Autodesk Fusion 360 part; units mm, degrees
sketch "Sketch1" plane through (0, 0, 0) normal (0, 0, 1) x (1, 0, 0)
  line L0 (0, 25) -> (64, 25)
  line L1 (64, 25) -> (64, -13)
  line L2 (64, -13) -> (0, -13)
  line L3 (0, -13) -> (0, 25)
  dimension "d1" = 64
  dimension "d2" = 38
extrude "Extrude1" add sketch "Sketch1" along normal blind 38
sketch "Sketch2" plane through (0, 0, 38) normal (0, 0, 1) x (1, 0, 0)
  line L0 (0, -13) -> (64, -13)
  line L1 (64, -13) -> (64, 25)
  line L2 (64, 25) -> (0, 25)
  line L3 (0, 25) -> (0, -13)
  line L4 (0, 25) -> (64, -13) construction
  line L5 (40.5159, 20.75) -> (23.4841, 20.75)
  line L6 (23.4841, 20.75) -> (14.9682, 6)
  line L7 (14.9682, 6) -> (23.4841, -8.75)
  line L8 (23.4841, -8.75) -> (40.5159, -8.75)
  line L9 (40.5159, -8.75) -> (49.0318, 6)
  line L10 (49.0318, 6) -> (40.5159, 20.75)
  circle A0 centre (32, 6) radius 11.75
  point P0 (32, 6)
  point P1 (32, 6)
  dimension "d5" = 14.75
  dimension "d8" = 23.5
extrude "Extrude2" cut sketch "Sketch2" against normal blind 8 contours L5 L6 L7 L8 L9 L10 | A0
extrude "Extrude3" cut sketch "Sketch2" against normal blind 52 contours A0
sketch "Sketch4" plane through (0, 0, 0) normal (-1, 0, 0) x (0, 0, 1)
  line L0 (0, 25) -> (0, -13)
  line L1 (0, -13) -> (38, -13)
  line L2 (38, -13) -> (38, 25)
  line L3 (38, 25) -> (0, 25)
  circle A0 centre (19, 6) radius 6.75 construction
  line L4 (2.0294, 22.9706) -> (35.9706, -10.9706) construction
  line L5 (19, 25) -> (19, -13) construction
  line L6 (2.0294, -10.9706) -> (35.9706, 22.9706) construction
  line L7 (2.0294, 22.9706) -> (11.3071, 6)
  line L8 (2.0294, 22.9706) -> (19, 13.6929)
  line L9 (35.9706, 22.9706) -> (19, 13.6929)
  line L10 (35.9706, 22.9706) -> (26.6929, 6)
  line L11 (35.9706, -10.9706) -> (26.6929, 6)
  line L12 (35.9706, -10.9706) -> (19, -1.6929)
  line L13 (2.0294, -10.9706) -> (19, -1.6929)
  line L14 (2.0294, -10.9706) -> (11.3071, 6)
  line L15 (19, 6) -> (2.0294, 22.9706) construction
  line L16 (8.5702, 16.4298) -> (10.5147, 18.3317) construction
  line L17 (9.5, 15.5) -> (11.6895, 17.6895) construction
  line L18 (11.3986, 13.6014) -> (14.1445, 16.3473) construction
  line L19 (12.8128, 12.1872) -> (15.9732, 15.3476) construction
  line L20 (9.5, 15.5) -> (28.5, 15.5) construction
  line L21 (28.5, 15.5) -> (28.5, -3.5) construction
  line L22 (28.5, -3.5) -> (9.5, -3.5) construction
  line L23 (9.5, -3.5) -> (9.5, 15.5) construction
  line L24 (28.5, 15.5) -> (9.5, -3.5) construction
  circle A1 centre (9.5, 15.5) radius 1
  circle A2 centre (28.5, 15.5) radius 1
  circle A3 centre (28.5, -3.5) radius 1
  circle A4 centre (9.5, -3.5) radius 1
  point P0 (19, 6)
  point P1 (12.8128, 12.1872)
  point P2 (11.3986, 13.6014)
  point P3 (9.5, 15.5)
  point P4 (8.5702, 16.4298)
  point P5 (14.227, 10.773)
  point P6 (28.5, 15.5)
  point P7 (9.5, -3.5)
  point P8 (28.5, -3.5)
  dimension "d11" = 13.5
  dimension "d12" = 48
  dimension "d13" = 48
  dimension "d33" = 19
  dimension "d34" = -19
  dimension "d35" = 2
  dimension "d36" = 2
  dimension "d37" = 2
  dimension "d38" = 2
extrude "Extrude4" cut sketch "Sketch4" against normal blind 3 contours L7 L8 L9 L10 L11 L12 L13 L14 | A1 | A2 | A3 | A4
fillet "Fillet1" radius 3 2 edges at (32, 25, 0) (32, -13, 0)
fillet "Fillet2" radius 3 2 edges at (32, 25, 38) (32, -13, 38)
sketch "Sketch5" plane through (64, 0, 0) normal (1, 0, 0) x (0, 0, -1)
  arc A0 (-38, -10) -> (-35, -13) centre (-35, -10) ccw
  line L0 (-35, -13) -> (-3, -13)
  arc A1 (-3, -13) -> (0, -10) centre (-3, -10) ccw
  line L1 (0, -10) -> (0, 22)
  arc A2 (0, 22) -> (-3, 25) centre (-3, 22) ccw
  line L2 (-3, 25) -> (-35, 25)
  arc A3 (-35, 25) -> (-38, 22) centre (-35, 22) ccw
  line L3 (-38, 22) -> (-38, -10)
  circle A4 centre (-19, 6) radius 11.25
  circle A5 centre (-19, 6) radius 4.5
  point P0 (-19, 25)
  point P1 (-19, -13)
  point P2 (-38, 6)
  point P3 (0, 6)
  point P4 (-19, 6)
  dimension "d20" = 22.5
  dimension "d21" = 9
extrude "Extrude5" cut sketch "Sketch5" against normal blind 18 contours A5
extrude "Extrude6" cut sketch "Sketch5" against normal blind 7 contours A4
extrude "Extrude7" cut sketch "Sketch4" against normal blind 4 contours L7 L8 L9 L10 L11 L12 L13 L14 | A1 | A2 | A3 | A4
extrude "Extrude8" cut sketch "Sketch4" against normal blind 7 contours A1 | A2 | A3 | A4
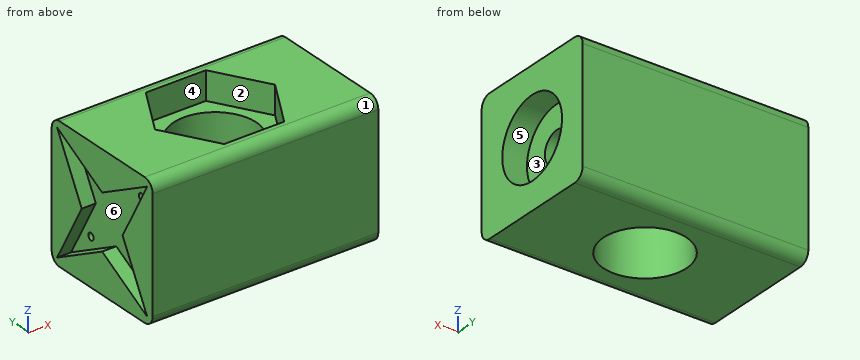
Geometry: final body of the model. Coordinates: model frame, mm. Face numbers are marked on the shaded views. A direction names the side the tool comes from. Coordinates: 2 decimals unless noted, no trailing zeros. Order: outer loops, then holes, each group sorted by start corner. A loop starts at its lowest first (then second) coordinate and runs counter-clockwise, first axis right, second up. Notation, with made-up numbers: M -23.75,51 L -12.75,51 A27 ccw -12.75,81 Z; hole C 64,1 d5. An arc over 180 degrees is marked long. Answer in a Markdown table with one row per item. Add a question column.
Q1. Section query A-A on x = 42.5. Return the cut outline in (y, z).
Q2. Section query D-D on x = 16. Return the cut outline in (y, z), and give its area (3 significant figures).
Q3. Line query: L1, parallel to Y at x = 5, z = 28.5; L2, parallel to Y at x = 32, z = 14; L3, parallel to X at y = 6.5, z = 7.5. Output: solid intervals per line, ascending.
Q4. Reachability of the marked faces 4, 5 and 6 from +Z, -Z, +X, -X, +Y, -Y: full face, straight path, thin tool, end or side. Return the list, or none.
Q5. Section query C-C on z = 9.5. Return the cut outline in (x, y), and give its area (3 significant figures).
Q6. Mould query, pull axis X, two halves, no side actions, for the marked faces 1, 2 and 3. Classes: released by +X, released by -X, zero draft, split by the parting line, or undercut.
Q7. Contact query for flat-ended pins moving along their axis: P1, Ø8, axis at x = 24, y = -8.5, coming from the +Z side; P2, Ø2, axis at y = -3, z = 9.5, coming from the -X side; P3, Ø11, axis at y = 1, z = 19.5, coming from the +X side. Output: stop coordinate, or through.
Q8. Section query B-B on y = 8. Return the cut outline in (x, z), and give its area (3 significant figures).
Completed:
| question | item | result |
|---|---|---|
| 1 | outline | M -13,3 A3 ccw -10,0 L 0.73,0 L 0.73,30 L -5.31,30 L -5.31,38 L -10,38 A3 ccw -13,35 Z; M 11.27,0 L 22,0 A3 ccw 25,3 L 25,35 A3 ccw 22,38 L 17.31,38 L 17.31,30 L 11.27,30 Z |
| 2 | outline | M -13,3 A3 ccw -10,0 L 22,0 A3 ccw 25,3 L 25,35 A3 ccw 22,38 L 7.79,38 L 7.79,30 L 4.21,30 L 4.21,38 L -10,38 A3 ccw -13,35 Z |
| 2 | area | 1,410 mm2 |
| 3 | L1 | y = -13 to -4.5, -2.5 to 14.5, 16.5 to 25 |
| 3 | L2 | y = -13 to -5.75, 17.75 to 25 |
| 3 | L3 | x = 0 to 20.26, 43.74 to 64 |
| 4 | face 4 | +Z |
| 4 | face 5 | +X |
| 4 | face 6 | -X |
| 5 | outline | M 0,-13 L 64,-13 L 64,-0.03 L 57,-0.03 L 57,12.03 L 64,12.03 L 64,25 L 0,25 L 0,18.89 L 4,18.89 L 4,16.5 L 7,16.5 L 7,14.5 L 4,14.5 L 4,9.31 L 0,9.31 L 0,2.69 L 4,2.69 L 4,-2.5 L 7,-2.5 L 7,-4.5 L 4,-4.5 L 4,-6.89 L 0,-6.89 Z; hole C 32,6 d23.5 |
| 5 | area | 1,830 mm2 |
| 6 | face 1 | zero draft |
| 6 | face 2 | undercut |
| 6 | face 3 | released by +X |
| 7 | P1 | stops at z = 38 |
| 7 | P2 | stops at x = 4 |
| 7 | P3 | stops at x = 57 |
| 8 | outline | M 0,0 L 20.42,0 L 20.42,30 L 16.12,30 L 16.12,38 L 0,38 L 0,27.79 L 4,27.79 L 4,10.21 L 0,10.21 Z; M 43.58,0 L 64,0 L 64,7.93 L 57,7.93 L 57,14.97 L 46,14.97 L 46,23.03 L 57,23.03 L 57,30.07 L 64,30.07 L 64,38 L 47.88,38 L 47.88,30 L 43.58,30 Z |
| 8 | area | 1,170 mm2 |
